Here's how the part is built. I have some questions about the finished solid (model axes, mm). A direction names the side the tool comes from. Round coordinates to 2 decimals unless told otherwise and drop trailing zeros. Order: outer loops, then holes, each group sorted by start corner. A loop starts at its lowest first (then second) coordinate and runs counter-clockwise, first axis right, second up. Notation, with made-up numbers: (46, 29) - (50, 29) arc R12 cw to (50, 50) - close; hole circle Ø7 at (80, 61). An arc over 180 degrees is marked (long way). Answer as a JSON object with one key per item and string values.
```python
from build123d import *

# Parameters (mm, degrees)
F1_DEPTH = 63.5
F0_W     = 25.4
F0_H     = 19.05
F2_DEPTH = 25.4
F3_DEPTH = 7.9375
F5_R     = 6.35


# Not quite as in the source:
# - a feature names something its author has since deleted; it is built from what else it names


with BuildPart() as f1:
    # F0 (on Front) → F1 (new body, symmetric)
    with BuildSketch(Plane.XZ):
        Polygon((41.275, -9.525), (41.275, 9.525), (22.225, 9.525), (-41.275, 9.525), (-41.275, -9.525), align=None)
    extrude(amount=F1_DEPTH, both=True)

    # F0 (on Front) → F2 (join, symmetric)
    with BuildSketch(Plane.XZ):
        with BuildLine():
            Line((22.225, 9.525), (41.275, 9.525))
            Line((41.275, 9.525), (41.275, 27.0006215875))
            ThreePointArc((41.275, 27.0006215875), (45.9656588405, 38.2667716764), (57.2656945294, 42.8752))
            Line((57.2656945294, 42.8752), (60.325, 42.8752))
            Line((60.325, 42.8752), (60.325, 61.9252))
            Line((60.325, 61.9252), (56.9783966597, 61.9252))
            add(Edge.make_bspline(
                [(55.5906283852, 61.8907919104), (56.0567092962, 61.9071657032), (56.5193514661, 61.918664428), (56.9783966597, 61.9252)],
                knots=[109.9767617242, 109.9767617242, 109.9767617242, 109.9767617242, 111.3530911794, 111.3530911794, 111.3530911794, 111.3530911794], degree=3))
            ThreePointArc((55.5906283852, 61.8907919104), (31.9089948829, 51.1387094503), (22.225, 27.0006215875))
            Line((22.225, 27.0006215875), (22.225, 9.525))
        make_face()
        with Locations((73.025, 52.4002)):
            Rectangle(F0_W, F0_H)
    extrude(amount=F2_DEPTH, both=True)

    # F0 (on Front) → F3 (join, symmetric)
    with BuildSketch(Plane.XZ):
        with BuildLine():
            Line((-41.275, 9.525), (22.225, 9.525))
            Line((22.225, 9.525), (22.225, 27.0006215875))
            ThreePointArc((22.225, 27.0006215875), (31.9089948829, 51.1387094503), (55.5906283852, 61.8907919104))
            add(Edge.make_bspline(
                [(-41.275, 9.525), (-40.8507124628, 28.1470359497), (18.3480415197, 60.5824302397), (55.5906283852, 61.8907919104)],
                knots=[0, 0, 0, 0, 109.9767617242, 109.9767617242, 109.9767617242, 109.9767617242], degree=3))
        make_face()
    extrude(amount=F3_DEPTH, both=True)

    # F0 (on Front) → F4 (revolve)
    with BuildSketch(Plane.XZ):
        Polygon((85.725, 61.9252), (85.725, 42.8752), (85.725, 38.1), (111.125, 38.1), (111.125, 66.675), (85.725, 66.675), align=None)
    revolve(axis=Axis((85.725, 0, 52.3875), (0, 0, 1)))

    # F5
    f5_edges = [f1.edges().sort_by_distance(p)[0] for p in [
        (-41.275, -63.5, 0),
        (41.275, -63.5, 0),
        (41.275, 63.5, 0),
        (-41.275, 63.5, 0),
    ]]
    fillet(f5_edges, radius=F5_R)


solid = f1.part
```
1. For P1, Ø12, axis at y = -16, z = 43, coming from the -X side; P2, Ø4, axis at x = 28, z = 57.5, coming from the -Y side; P3, Ø15.5, axis at x = 22.5, z = 27, coming from the -Y side, each with a flat end and sliding along its axis, tell me the tip position at first contact or that it passes through.
Responses:
{"P1": "x = 23.69", "P2": "y = -7.94", "P3": "y = -25.4"}
2. Imagine slicing it at B-B (y = 45.5). List the corners of the cut face in (x, z) for me (3 decimals), plus the area to 3 significant figures.
Responses:
{"outline": "(-41.275, -9.525) - (41.275, -9.525) - (41.275, 9.525) - (-41.275, 9.525) - close", "area": "1,570 mm2"}
3. Thinking about a two-plate mould opening in X: for faces 1 (the face through (45.8, -0.4, 38.1)), 2 (the face through (39.464, -61.59, 0.133)), 3 (the face through (60, 0, 61.925)), which applies, pulls with the +X half, pulls with the -X half, needs draft (parallel to the pull), parting line crosses it, or undercut?
Responses:
{"face 1": "undercut", "face 2": "pulls with the +X half", "face 3": "needs draft"}
4. For faces 4 (the face through (22.225, -17, 18)), 5 (the face through (46, 25.4, 42)), 6 (the face through (60, 2, 42.875)), which set-ups out of +Z, -Z, +X, -X, +Y, -Y let a thin tool reach every point of the face, with its end or its side?
Responses:
{"face 4": "+Z, -X, -Y", "face 5": "+Z, +X, -X, +Y", "face 6": "-Z"}
5. Imagine slicing it at A-A (z = 5). List the corners of the cut face in (x, y) for me (3 decimals), plus the area to 3 significant figures.
Responses:
{"outline": "(-41.275, -57.15) arc R6.35 ccw to (-34.925, -63.5) - (34.925, -63.5) arc R6.35 ccw to (41.275, -57.15) - (41.275, 57.15) arc R6.35 ccw to (34.925, 63.5) - (-34.925, 63.5) arc R6.35 ccw to (-41.275, 57.15) - close", "area": "10,400 mm2"}
6. Imagine slicing it at C-C (x = 96). List the corners of the cut face in (y, z) for me (3 decimals).
Responses:
{"outline": "(-23.229, 38.1) - (23.229, 38.1) - (23.229, 66.675) - (-23.229, 66.675) - close"}
7. If I drill on L1, parallel to Y at x = 53, z = 61; L2, parallel to Z at x = 63.5, y = 25; L3, parallel to Y at x = -19.5, z = 24, over which ranges is the centre line in solid material (lowest first)? Write a range as [from, to].
Responses:
{"L1": "[-25.4, 25.4]", "L2": "[42.88, 61.93]", "L3": "[-7.94, 7.94]"}
